```python
from build123d import *

# Parameters (mm, degrees)
F1_W     = 114.3
F1_H     = 190.5
F2_DEPTH = 118.11
F3_R     = 3.96875
F4_DEPTH = 118.11
F5_W     = 38.1
F5_H     = 114.3
F6_DEPTH = 118.11
F7_R     = 0.254


with BuildPart() as f2:
    # F1 (on Front) → F2 (new body)
    with BuildSketch(Plane.XZ):
        Rectangle(F1_W, F1_H)
    extrude(amount=-F2_DEPTH)

    # F3 (on face) → F4 (cut)
    with BuildSketch(Plane.XZ):
        with Locations((-46.0375, 84.1375)):
            Circle(F3_R)
        with Locations((46.0375, 84.1375)):
            Circle(F3_R)
        with Locations((-46.0375, -84.1375)):
            Circle(F3_R)
        with Locations((46.0375, -84.1375)):
            Circle(F3_R)
    extrude(amount=-F4_DEPTH, mode=Mode.SUBTRACT)

    # F5 (on face) → F6 (cut)
    with BuildSketch(Plane.XZ):
        Rectangle(F5_W, F5_H)
    extrude(amount=-F6_DEPTH, mode=Mode.SUBTRACT)

    # F7
    f7_edges = [f2.edges().sort_by_distance(p)[0] for p in [
        (-19.05, 59.055, 57.15),
        (19.05, 59.055, 57.15),
        (19.05, 59.055, -57.15),
        (-19.05, 59.055, -57.15),
    ]]
    fillet(f7_edges, radius=F7_R)


solid = f2.part
```
Geometry check sheet. Reference: the model listing, model coordinates, mm. A direction names the side the tool comes from. Round coordinates to 2 decimals unless told otherwise and drop trailing zeros. Order: outer loops, then holes, each group sorted by start corner. A loop starts at its lowest first (then second) coordinate and runs counter-clockwise, first axis right, second up. Notation, with made-up numbers: (65, 18.5) -> (102, 18.5) arc R26 cw to (102, 34.5) -> close; hole circle Ø10 at (35, 20.25). An arc over 180 degrees is marked (long way). Return JSON: item names as keys, results as strings. Group by question number.
Q1. Tool access check on faces 1 (the flat face through (25, 0, 1)), 2 (the flat face through (-19.05, 58, -1)). Record the directions out of +Z, -Z, +X, -X, +Y, -Y that give a thin tool (end or side, any length) a straight path to the whole face; none if there is none.
Q2. Section check A-A, the plane x = -2.5. Record the boundary of the cut face in (y, z), plus the area to 3 significant figures.
Q3. Section check C-C, the plane y = 54.5. Record the boundary of the cut face in (x, z), plus the area to 3 significant figures.
Q4. Section check D-D, the plane x = 47. Record the boundary of the cut face in (y, z), plus the area to 3 significant figures.
Q5. Release check for a two-part mould opening along X. For faces 3 (the flat face through (-1, 58, 95.25)), 4 (the flat face through (19.05, 58, -1)), 5 (the cylindrical face through (49.823, 58.228, 85.33)), 6 (the flat face through (57.15, 58, -1)) record: released by +X, released by -X, zero draft, split by the parting line, or undercut.
Q6. Section check B-B, the plane z = -4. Record the boundary of the cut face in (x, y), plus the area to 3 significant figures.
Q7. Material ranges on probe 1 along Z at (x, y) = (46, 60); probe 2 along X at (y, z) = (55.5, -54.5); probe 3 along Z at (x, y) = (-11, 110.5), recorded low to high. Write a range as from..to.
Numbers:
{
 "1": {"face 1": "+Z, -Z, +X, -X, -Y", "face 2": "+Y, -Y"},
 "2": {"outline": "(0, -95.25) -> (118.11, -95.25) -> (118.11, -57.15) -> (0, -57.15) -> close; (0, 57.15) -> (118.11, 57.15) -> (118.11, 95.25) -> (0, 95.25) -> close", "area": "9,000 mm^2"},
 "3": {"outline": "(-57.15, -95.25) -> (57.15, -95.25) -> (57.15, 95.25) -> (-57.15, 95.25) -> close; hole circle Ø7.94 at (-46.04, -84.14); hole circle Ø7.94 at (-46.04, 84.14); hole (-19.05, -56.9) arc R0.25 ccw to (-18.8, -57.15) -> (18.8, -57.15) arc R0.25 ccw to (19.05, -56.9) -> (19.05, 56.9) arc R0.25 ccw to (18.8, 57.15) -> (-18.8, 57.15) arc R0.25 ccw to (-19.05, 56.9) -> close; hole circle Ø7.94 at (46.04, -84.14); hole circle Ø7.94 at (46.04, 84.14)", "area": "17,200 mm^2"},
 "4": {"outline": "(0, -95.25) -> (118.11, -95.25) -> (118.11, -87.99) -> (0, -87.99) -> close; (0, -80.29) -> (118.11, -80.29) -> (118.11, 80.29) -> (0, 80.29) -> close; (0, 87.99) -> (118.11, 87.99) -> (118.11, 95.25) -> (0, 95.25) -> close", "area": "20,700 mm^2"},
 "5": {"face 3": "zero draft", "face 4": "undercut", "face 5": "undercut", "face 6": "released by +X"},
 "6": {"outline": "(-57.15, 0) -> (-19.05, 0) -> (-19.05, 118.11) -> (-57.15, 118.11) -> close; (19.05, 0) -> (57.15, 0) -> (57.15, 118.11) -> (19.05, 118.11) -> close", "area": "9,000 mm^2"},
 "7": {"probe 1": "-95.25..-88.11, -80.17..80.17, 88.11..95.25", "probe 2": "-57.15..-19.05, 19.05..57.15", "probe 3": "-95.25..-57.15, 57.15..95.25"}
}
